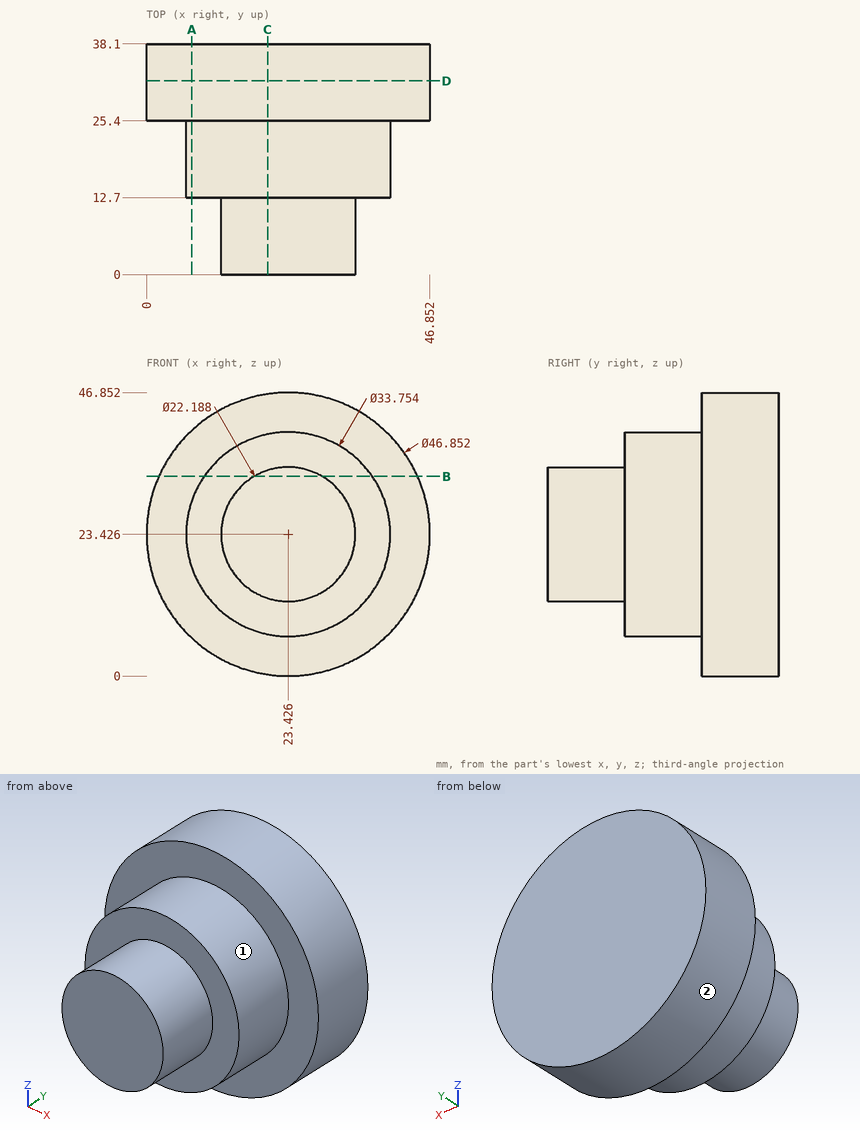
For this review, use the dimensioned drawing (mm, ordinates from the lowest corner) and the shaded views. A direction names the side the tool comes from. Round coordinates to 2 decimals unless told otherwise and drop trailing zeros. Order: outer loops, then holes, each group sorted by start corner. A loop starts at its lowest first (then second) coordinate and runs counter-clockwise, first axis right, second up. Notation, with made-up numbers: (0.25, 86.25) -> (54.25, 86.25) arc R8 cw to (54.25, 98.25) -> close; hole circle Ø5 at (37, -19.75). An arc over 180 degrees is marked (long way). Write item = value, one per line. Start each with the question number.
Item 1: For the marked faces 1 and 2, list the 3-axis set-ups (+Z, -Z, +X, -X, +Y, -Y) from which the entire face can be reached by the end or side of a thin tool; tool diameter is ignored.
Item 2: Clearance check with flat-ended pins moving along their axes: pin 1 Ø6 at (y, z) = (20.5, 22.5) entering from +X; pin 2 Ø4 at (x, y) = (24.5, 31) entering from -Z; pin 3 Ø1 at (x, y) = (22, 22.5) entering from -Z (1 decimal). State where each tip first meets the part, or that it passes through.
Item 3: For line 1 along X through (y, z) = (24.5, 23) (1 decimal); line 2 along Y through (x, z) = (25, 35); line 3 along Y through (x, z) = (44, 29.5), list the stretches that pass through material, from the lowest coordinate up.
Item 4: Consider section A-A on x = 7.5. Write out the cut boundary in (y, z).
Item 5: Consider section C-C on x = 20. Write out the cut boundary in (y, z) (1 decimal).
Item 6: Consider section B-B on z = 33. Write out the cut boundary in (x, y) (1 decimal), plus the area to 3 significant figures.
Item 7: Consider section D-D on y = 32. Write out the cut boundary in (x, z).
Conclusion:
q1.face_1 = -Y
q1.face_2 = +Y, -Y
q2.pin_1 = 40.3
q2.pin_2 = 0
q2.pin_3 = 6.6
q3.line_1 = 6.6 to 40.3
q3.line_2 = 12.7 to 38.1
q3.line_3 = 25.4 to 38.1
q4.outline = (12.7, 17.84) -> (25.4, 17.84) -> (25.4, 6.25) -> (38.1, 6.25) -> (38.1, 40.61) -> (25.4, 40.61) -> (25.4, 29.01) -> (12.7, 29.01) -> close
q5.outline = (0, 12.9) -> (12.7, 12.9) -> (12.7, 6.9) -> (25.4, 6.9) -> (25.4, 0.3) -> (38.1, 0.3) -> (38.1, 46.6) -> (25.4, 46.6) -> (25.4, 40) -> (12.7, 40) -> (12.7, 34) -> (0, 34) -> close
q6.outline = (2, 25.4) -> (9.5, 25.4) -> (9.5, 12.7) -> (17.8, 12.7) -> (17.8, 0) -> (29, 0) -> (29, 12.7) -> (37.3, 12.7) -> (37.3, 25.4) -> (44.8, 25.4) -> (44.8, 38.1) -> (2, 38.1) -> close
q6.area = 1,040 mm2
q7.outline = circle Ø46.85 at (23.43, 23.43)
